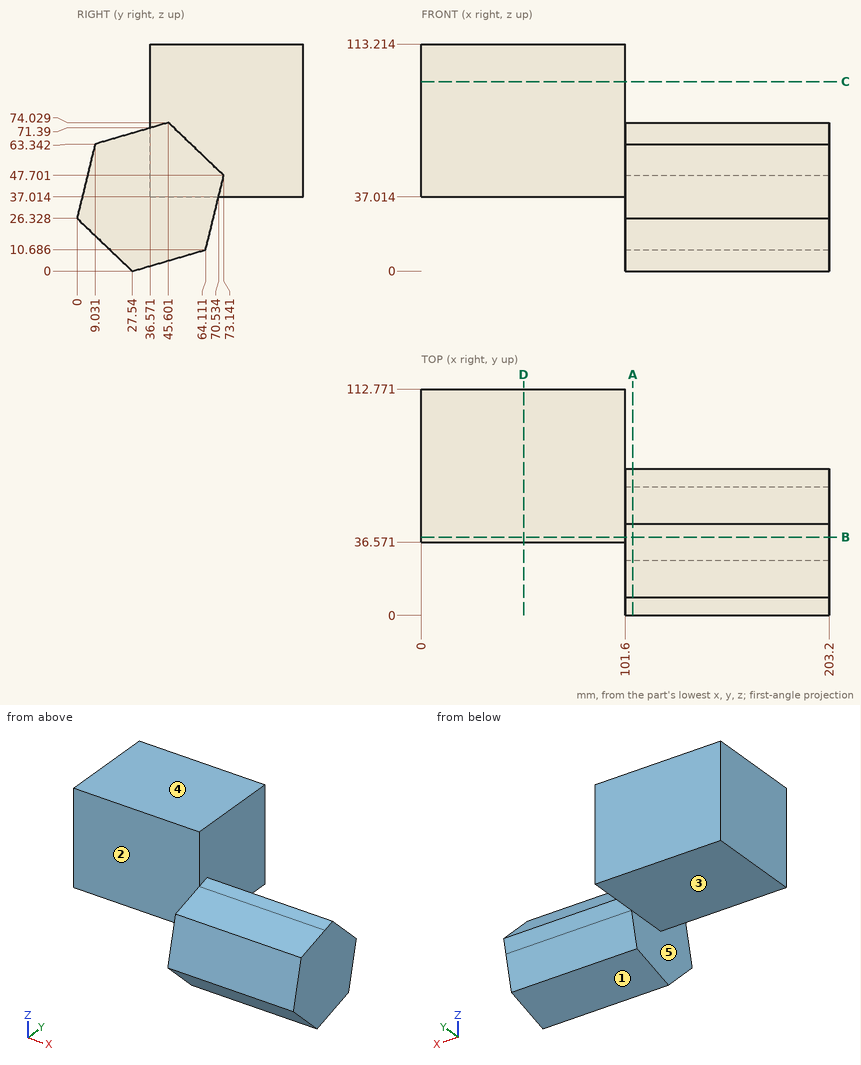
Here's the drawing with two shaded views (mm, measured from the low corner). I have some questions. A direction names the side the tool comes from. Give positions to 0.01 mm unless a question says otherwise; leave off trailing zeros. Order: outer loops, then holes, each group sorted by start corner. A loop starts at its lowest first (then second) coordinate and runs counter-clockwise, first axis right, second up. Notation, with made-up numbers: (54.5, -16) -> (105.5, -16) arc R26 cw to (105.5, 15) -> close; hole circle Ø5 at (45, 67). An arc over 180 degrees is marked (long way). Use a Markdown table: item, result. Add a question column.
Item 1: Imagine slicing it at A-A on x = 105.5. Please give me the cut outline in (y, z) (1 decimal).
Item 2: Imagine slicing it at C-C on z = 94.5. Please give me the cut outline in (x, y).
Item 3: If we mould it in two halves opening along Z, with no side actions, what happens to the marked faces 3, 4 and 5? For each: pulls with the +Z half, pulls with the -Z half, needs draft (parallel to the pull), parting line crosses it, or undercut.
Item 4: For the marked faces 1 and 2, which set-ups out of +Z, -Z, +X, -X, +Y, -Y let a thin tool reach every point of the face, with its end or its side?
Item 5: Imagine slicing it at B-B on y = 39. Please give me the cut outline in (x, z) (1 decimal), plus the area to 3 significant figures.
Item 6: Will these pins go through, and if not, where does the flat tip stop? pin 1 (1.5 mm diameter, centred on y = 74.5, z = 65.5, fed in from +X); pin 2 (1 mm diameter, centred on x = 119.5, z = 50.5, fed in from +Y) (1 decimal); pin 3 (2 mm diameter, centred on x = 123, y = 45, fed in from -Z).
Item 7: I need wall thicknesses on line 1 (Z direction, x = 49.5, y = 73) (1 decimal); line 2 (X direction, y = 10.5, z = 59); line 3 (X direction, y = 89, z = 92). Which ranges of each line are inside material? Lowest first, please.
Item 8: Imagine slicing it at D-D on x = 51. Please give me the cut outline in (y, z) (1 decimal), plus the area to 3 significant figures.
Data:
| question | item | result |
|---|---|---|
| 1 | outline | (0, 26.3) -> (27.5, 0) -> (64.1, 10.7) -> (73.1, 47.7) -> (45.6, 74) -> (9, 63.3) -> close |
| 2 | outline | (0, 36.57) -> (101.6, 36.57) -> (101.6, 112.77) -> (0, 112.77) -> close |
| 3 | face 3 | pulls with the -Z half |
| 3 | face 4 | pulls with the +Z half |
| 3 | face 5 | needs draft |
| 4 | face 1 | -Z, +X, -X, +Y |
| 4 | face 2 | +Z, -Z, -X, -Y |
| 5 | outline | (0, 37) -> (101.6, 37) -> (101.6, 3.3) -> (203.2, 3.3) -> (203.2, 72.1) -> (101.6, 72.1) -> (101.6, 113.2) -> (0, 113.2) -> close |
| 5 | area | 14,700 mm² |
| 6 | pin 1 | stops at x = 101.6 |
| 6 | pin 2 | stops at y = 70.7 |
| 6 | pin 3 | stops at z = 4.81 |
| 7 | line 1 | z = 37 to 113.2 |
| 7 | line 2 | x = 101.6 to 203.2 |
| 7 | line 3 | x = 0 to 101.6 |
| 8 | outline | (36.6, 37) -> (112.8, 37) -> (112.8, 113.2) -> (36.6, 113.2) -> close |
| 8 | area | 5,810 mm² |
